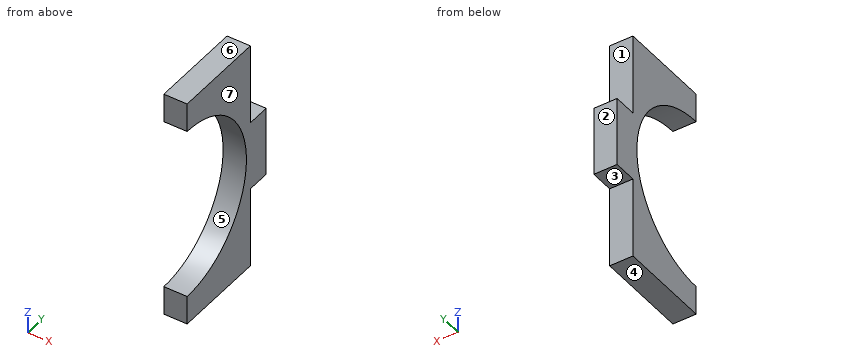
```python
from build123d import *

# Parameters (mm, degrees)
BOSS_EXTRUDE1_DEPTH = 3.175


with BuildPart() as part:
    # Sketch1 → Boss-Extrude1 (new body)
    with BuildSketch(Plane(origin=(0, 0, 0), x_dir=(0, 0, -1), z_dir=(1, 0, 0))):
        with BuildLine():
            Line((11.1125, 12.7), (11.1125, 15.875))
            Line((11.1125, 15.875), (20.6375, 15.875))
            Line((20.6375, 15.875), (20.6375, 12.7))
            Line((20.6375, 12.7), (31.75, 12.7))
            Line((31.75, 12.7), (31.75, 0))
            Line((31.75, 0), (27.78125, 0))
            ThreePointArc((27.78125, 0), (15.875, 11.90625), (3.96875, 0))
            Line((3.96875, 0), (0, 0))
            Line((0, 0), (0, 12.7))
            Line((0, 12.7), (11.1125, 12.7))
        make_face()
    extrude(amount=BOSS_EXTRUDE1_DEPTH)


solid = part.part
```
Here's how the part is built. I have some questions about the finished solid (model axes, mm). Face numbers are marked on the shaded views. A direction names the side the tool comes from. Coordinates: 2 decimals unless noted, no trailing zeros. Loops run counter-clockwise (first coordinate to the right, second up) from the corner with the lowest first, then second, coordinate; pieces in that order, holes last. Notation, with made-up numbers: M 7.25,-27.75 L 41.25,-27.75 A29 cw 41.25,9.25 Z; hole C -2,51.25 d8. An arc over 180 degrees is marked long. One line per item, written item: value.
1. Will this pin go through, and if not, where does the flat tip stop? pin 1 Ø1 at (x, z) = (1.5, -26.5) entering from +Y.
Geometry says:
pin 1: stops at y = 12.7
2. Imagine slicing it at A-A (y = 11). List the corners of the cut face in (x, z) for me (3 decimals), and give its area (3 significant figures).
Geometry says:
outline: M 0,-31.75 L 3.175,-31.75 L 3.175,-20.431 L 0,-20.431 Z; M 0,-11.319 L 3.175,-11.319 L 3.175,0 L 0,0 Z
area: 71.9 mm2
3. Imagine slicing it at C-C (z = -28.5). List the corners of the cut face in (x, y) for me (3 decimals), and give its area (3 significant figures).
Geometry says:
outline: M 0,0 L 3.175,0 L 3.175,12.7 L 0,12.7 Z
area: 40.3 mm2
4. Imagine slicing it at D-D (y = 14.25). List the corners of the cut face in (x, z) for me (1 decimal).
Geometry says:
outline: M 0,-20.6 L 3.2,-20.6 L 3.2,-11.1 L 0,-11.1 Z
5. Thinking about a two-plate mould opening in Z: for the marked faces 4, 5, 6 and 7, which applies, +Z half, -Z half, draft (parallel to the pull), parting line (faces both ways), or undercut?
Geometry says:
face 4: -Z half
face 5: undercut
face 6: +Z half
face 7: draft
6. On a 3-axis mill with a long thin cutter (end or side, diameter ignored), from which of +Z, -Z, +X, -X, +Y, -Y can I reach the whole of each face in a straight line? I mean the marked faces 1, 2 and 3. Say none if no direction works.
Geometry says:
face 1: +Z, +X, -X, +Y
face 2: +Z, -Z, +X, -X, +Y
face 3: -Z, +X, -X, +Y
7. Please list where these lines run through material, in increasing order: probe 1 along Y at (x, z) = (2.85, -30); probe 2 along Z at (x, y) = (0.8, 14.5); probe 3 along Z at (x, y) = (0.35, 2.75).
Geometry says:
probe 1: y = 0 to 12.7
probe 2: z = -20.64 to -11.11
probe 3: z = -31.75 to -27.46, -4.29 to 0
